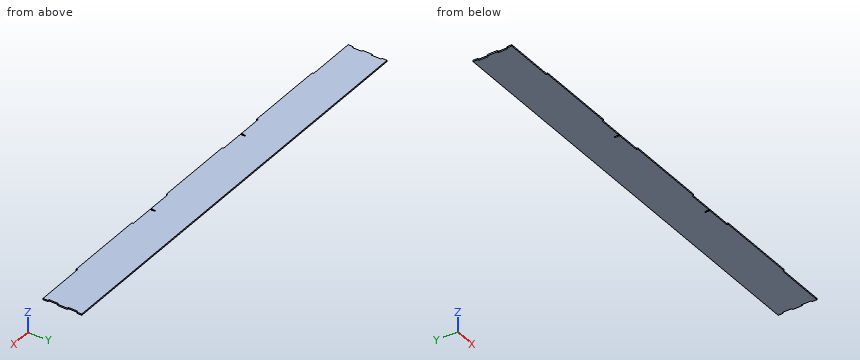
```python
from build123d import *

# Parameters (mm, degrees)
SALIENTE_EXTRUIR1_DEPTH = 5
CROQUIS2_W              = 5
CROQUIS2_H              = 35
CORTAR_EXTRUIR1_DEPTH   = 5
CORTAR_EXTRUIR2_DEPTH   = 10


with BuildPart() as part:
    # Croquis1 → Saliente-Extruir1 (new body)
    with BuildSketch(Plane.XY):
        Polygon((0, 145), (0, 0), (183.734642654, 0), (185, 0), (185, -5), (485, -5), (485, 0), (670, 0), (670, -5), (970, -5), (970, 0), (1155, 0), (1155, -5), (1455, -5), (1455, 0), (1640, 0), (1640, 145), align=None)
    extrude(amount=SALIENTE_EXTRUIR1_DEPTH)

    # Croquis2 → Cortar-Extruir1 (cut)
    with BuildSketch(Plane.XY.offset(5)):
        with Locations((1637.5, 108.75)):
            Rectangle(CROQUIS2_W, CROQUIS2_H)
        with Locations((1637.5, 36.25)):
            Rectangle(CROQUIS2_W, CROQUIS2_H)
        with Locations((2.5, 36.25)):
            Rectangle(CROQUIS2_W, CROQUIS2_H)
        with Locations((2.5, 108.75)):
            Rectangle(CROQUIS2_W, CROQUIS2_H)
    extrude(amount=-CORTAR_EXTRUIR1_DEPTH, mode=Mode.SUBTRACT)

    # Croquis3 → Cortar-Extruir2 (cut)
    with BuildSketch(Plane.XY.offset(5)):
        Polygon((579.3, 0), (575.7, 0), (575.7, 5), (573.9, 5), (573.9, 8.2), (575.7, 8.2), (575.7, 17.2), (579.3, 17.2), (579.3, 8.2), (581.1, 8.2), (581.1, 5), (579.3, 5), align=None)
        Polygon((1064.3, 8.2), (1064.3, 17.2), (1060.7, 17.2), (1060.7, 8.2), (1058.9, 8.2), (1058.9, 5), (1060.7, 5), (1060.7, 0), (1064.3, 0), (1064.3, 5), (1066.1, 5), (1066.1, 8.2), align=None)
    extrude(amount=-CORTAR_EXTRUIR2_DEPTH, mode=Mode.SUBTRACT)


solid = part.part
```
Check sheet for the modelled part. Datum: model origin and axes. Units: mm. Round coordinates to 2 decimals unless told otherwise and drop trailing zeros. Loops run counter-clockwise (first coordinate to the right, second up) from the corner with the lowest first, then second, coordinate; pieces in that order, holes last. Notation, with made-up numbers: (43.25, 17.25) - (64.25, 17.25) arc R20 ccw to (64.25, 34.25) - close; hole circle Ø7 at (22.5, -4). An arc over 180 degrees is marked (long way). Answer as a JSON object with one key per item and string values. Group by question number.
Q1. Sectioned sample at A-A, the plane x = 1538.5. Enter the section's corners in (y, z), plus the area to 3 significant figures.
Q2. Scan lines: line 1 along X through (y, z) = (5.5, 1.4); line 2 along X through (y, z) = (4.5, 1.3); line 3 along X through (y, z) = (31.5, 4.2). Record each from-to range of solid material in increasing order. Write a range as [from, to].
Q3. Gauge pin test, flat ends, axial feed: P1, Ø1.5, axis at y = 33.5, z = 1.5, coming from the -X side; P2, Ø1.1, axis at x = 577.5, z = 3, coming from the -Y side; P3, Ø2.5, axis at x = 3, z = 2, coming from the -Y side. Record the tip position at first contact, or that the pin passes through.
Solution:
{
 "1": {"outline": "(0, 0) - (145, 0) - (145, 5) - (0, 5) - close", "area": "725 mm²"},
 "2": {"line 1": "x = [0, 573.9], [581.1, 1058.9], [1066.1, 1640]", "line 2": "x = [0, 575.7], [579.3, 1060.7], [1064.3, 1640]", "line 3": "x = [5, 1635]"},
 "3": {"P1": "stops at x = 5", "P2": "stops at y = 17.2", "P3": "stops at y = 0"}
}
